from build123d import *

# Parameters (mm, degrees)
SKETCH1_R           = 133.35
SKETCH1_R_2         = 110.49
BOSS_EXTRUDE1_DEPTH = 20.32
FILLET1_R           = 5.08
FILLET4_R           = 5.08
FILLET5_R           = 5.08
FILLET6_R           = 5.08
SKETCH2_R           = 25.4
BOSS_EXTRUDE2_DEPTH = 12.7
SKETCH3_R           = 11.43
BOSS_EXTRUDE3_DEPTH = 381


with BuildPart() as part:
    # Sketch1 → Boss-Extrude1 (new body)
    with BuildSketch(Plane.XY):
        Circle(SKETCH1_R)
        Circle(SKETCH1_R_2, mode=Mode.SUBTRACT)
    extrude(amount=BOSS_EXTRUDE1_DEPTH)

    # Fillet1
    fillet1_edges = [part.edges().sort_by_distance(p)[0] for p in [
        (-133.35, 0, 20.32),
    ]]
    fillet(fillet1_edges, radius=FILLET1_R)

    # Fillet4
    fillet4_edges = [part.edges().sort_by_distance(p)[0] for p in [
        (-133.35, 0, 0),
    ]]
    fillet(fillet4_edges, radius=FILLET4_R)

    # Fillet5
    fillet5_edges = [part.edges().sort_by_distance(p)[0] for p in [
        (-110.49, 0, 20.32),
    ]]
    fillet(fillet5_edges, radius=FILLET5_R)

    # Fillet6
    fillet6_edges = [part.edges().sort_by_distance(p)[0] for p in [
        (-110.49, 0, 0),
    ]]
    fillet(fillet6_edges, radius=FILLET6_R)



with BuildPart() as body_2:
    # Sketch2 → Boss-Extrude2 (new body)
    with BuildSketch(Plane.XY.offset(20.32)):
        with BuildLine():
            add(Edge.make_bspline(
                [(111.995773379, 28.519671196), (108.395461325, 33.640925655), (103.465758881, 38.766955506)],
                knots=[0.86323948, 0.86323948, 0.86323948, 1, 1, 1], degree=2))
            Line((103.465758881, 38.766955506), (17.465361403, 18.442373791))
            ThreePointArc((17.465361403, 18.442373791), (23.332168562, 10.038421698), (25.4, 0))
            ThreePointArc((25.4, 0), (23.332168562, -10.038421698), (17.465361403, -18.442373791))
            Line((17.465361403, -18.442373791), (104.480917214, -35.941313806))
            add(Edge.make_bspline(
                [(104.480917214, -35.941313806), (109.199570697, -30.926942984), (112.628608991, -25.907939648)],
                knots=[0, 0, 0, 0.134699054, 0.134699054, 0.134699054], degree=2))
            ThreePointArc((112.628608991, -25.907939648), (114.832297811, -13.037188327), (115.57, 0))
            ThreePointArc((115.57, 0), (114.672962004, 14.37138425), (111.995773379, 28.519671196))
        make_face()
        with BuildLine():
            ThreePointArc((-17.465361403, 18.442373791), (0, 25.4), (17.465361403, 18.442373791))
            Line((17.465361403, 18.442373791), (41.120888712, 102.55297466))
            add(Edge.make_bspline(
                [(33.408134269, 110.6359863), (37.257292789, 107.035833442), (41.120888712, 102.55297466)],
                knots=[0.898413925, 0.898413925, 0.898413925, 1, 1, 1], degree=2))
            ThreePointArc((33.408134269, 110.6359863), (3.618968694, 115.513323758), (-26.417084957, 112.510277408))
            add(Edge.make_bspline(
                [(-33.5455644, 105.274570572), (-29.987921782, 109.295772293), (-26.417084957, 112.510277408)],
                knots=[0, 0, 0, 0.097113874, 0.097113874, 0.097113874], degree=2))
            Line((-33.5455644, 105.274570572), (-17.465361403, 18.442373791))
        make_face()
        with BuildLine():
            Line((41.120888883, -102.552974591), (17.465361403, -18.442373791))
            ThreePointArc((17.465361403, -18.442373791), (0, -25.4), (-17.465361403, -18.442373791))
            Line((-17.465361403, -18.442373791), (-33.545564575, -105.274570516))
            add(Edge.make_bspline(
                [(-33.545564575, -105.274570516), (-26.738144431, -110.571915765), (-19.922448027, -113.839891798)],
                knots=[0, 0, 0, 0.182948004, 0.182948004, 0.182948004], degree=2))
            ThreePointArc((-19.922448027, -113.839891798), (3.568860133, -115.514882753), (26.911965601, -112.392931306))
            add(Edge.make_bspline(
                [(26.911965601, -112.392931306), (34.011973832, -108.564945177), (41.120888883, -102.552974591)],
                knots=[0.810210618, 0.810210618, 0.810210618, 1, 1, 1], degree=2))
        make_face()
        with BuildLine():
            ThreePointArc((-17.465361403, -18.442373791), (-25.4, 0), (-17.465361403, 18.442373791))
            Line((-17.465361403, 18.442373791), (-103.453712161, 38.799092001))
            add(Edge.make_bspline(
                [(-111.872978372, 28.997613871), (-108.286344087, 33.895850119), (-103.453712161, 38.799092001)],
                knots=[0.869248391, 0.869248391, 0.869248391, 1, 1, 1], degree=2))
            ThreePointArc((-111.872978372, 28.997613871), (-115.56181287, 1.375611191), (-112.531537583, -26.326373643))
            add(Edge.make_bspline(
                [(-104.492035357, -35.908977246), (-109.115451856, -31.120100592), (-112.531537583, -26.326373643)],
                knots=[0, 0, 0, 0.128706822, 0.128706822, 0.128706822], degree=2))
            Line((-104.492035357, -35.908977246), (-17.465361403, -18.442373791))
        make_face()
        Circle(SKETCH2_R)
    extrude(amount=-BOSS_EXTRUDE2_DEPTH)


with BuildPart() as part_1:
    add(part.part)

    add(body_2.part)  # Boss-Extrude3 merges body 2
    # Sketch3 → Boss-Extrude3 (add)
    with BuildSketch(Plane.XY.offset(20.32)):
        Circle(SKETCH3_R)
    extrude(amount=BOSS_EXTRUDE3_DEPTH)


solid = part_1.part
Source: CAD feature listing. Evaluate the final solid. Frame: model axes, mm. A direction names the side the tool comes from. Give positions to 0.01 mm unless a question says otherwise; leave off trailing zeros. Loops run counter-clockwise (first coordinate to the right, second up) from the corner with the lowest first, then second, coordinate; pieces in that order, holes last. Notation, with made-up numbers: (-37.75, 47) -> (7.25, 47) arc R30 ccw to (7.25, 76) -> close; hole circle Ø3 at (35, 49.5). An arc over 180 degrees is marked (long way). Use a Markdown table: item, result. Add a question column.
1) First-contact query: pin 1 (6 mm diameter, centred on x = -46, y = 100.5, fed in from -Z); pin 2 (6 mm diameter, centred on x = -52, y = 27, fed in from +Z); pin 3 (1.5 mm diameter, centred on x = 5.5, z = 342.5, fed in from -Y). Flat tips, straight axial feed; report the tip coordinate or a pass-through.
2) Reachability of faces 1 (the face through (-2, 2, 7.62)), 2 (the face through (61.068, 28.747, 14.059)), 3 (the face through (-115, 20, 0)) from +Z, -Z, +X, -X, +Y, -Y: full face, straight path, thin tool, end or side. Return the list, or none.
3) Pull-direction query (X, two-part tool) for faces 4 (the face through (-25.393, -61.251, 14.059)), 5 (the face through (10.902, 3.433, 208.153)), 6 (the face through (-2, -27, 20.32)), 7 (the face through (29.128, 59.909, 14.059)); classes: +X half, -X half, draft (parallel to the pull), parting line (faces both ways), or undercut.
4) Section query C-C, the plane x = -58. Count the separate pieces of the cut face and the enclosed holes in it, then the cut area to 3 significant figures.
5) Line query: line 1 along Z through (x, y) = (-14.5, 91); line 2 along Z through (x, y) = (-78.5, -84.5); line 3 along Y through (x, z) = (0, 9). Output: solid intervals per line, ascending. Write a range as [from, to].
6) Section query A-A, the plane x = 0. Return the cut outline in (y, z).
Numbers:
| question | item | result |
|---|---|---|
| 1 | pin 1 | stops at z = 0.43 |
| 1 | pin 2 | stops at z = 20.32 |
| 1 | pin 3 | stops at y = -10.4 |
| 2 | face 1 | -Z |
| 2 | face 2 | +Z, -Z |
| 2 | face 3 | -Z, +X, -X, +Y, -Y |
| 3 | face 4 | undercut |
| 3 | face 5 | parting line |
| 3 | face 6 | draft |
| 3 | face 7 | undercut |
| 4 | separate pieces | 3 |
| 4 | enclosed holes | 0 |
| 4 | area | 1,700 mm2 |
| 5 | line 1 | z = [7.62, 20.32] |
| 5 | line 2 | z = [0.01, 20.31] |
| 5 | line 3 | y = [-133.35, 133.35] |
| 6 | outline | (-133.35, 5.08) arc R5.08 ccw to (-128.27, 0) -> (-115.57, 0) arc R5.08 ccw to (-110.49, 5.08) -> (-110.49, 7.62) -> (110.49, 7.62) -> (110.49, 5.08) arc R5.08 ccw to (115.57, 0) -> (128.27, 0) arc R5.08 ccw to (133.35, 5.08) -> (133.35, 15.24) arc R5.08 ccw to (128.27, 20.32) -> (11.43, 20.32) -> (11.43, 401.32) -> (-11.43, 401.32) -> (-11.43, 20.32) -> (-128.27, 20.32) arc R5.08 ccw to (-133.35, 15.24) -> close |
